```python
from build123d import *

# Parameters (mm, degrees)
F0_W     = 50
F0_H     = 50
F1_DEPTH = 50
F2_R     = 12.5
F3_DEPTH = 213.370338
F4_R     = 10
F5_R     = 12.5
F6_DEPTH = 50
F7_R     = 12.5
F8_DEPTH = 50


with BuildPart() as f1:
    # F0 (on Top) → F1 (new body)
    with BuildSketch(Plane.XY):
        Rectangle(F0_W, F0_H)
    extrude(amount=F1_DEPTH)

    # F2 (on Top) → F3 (cut)
    with BuildSketch(Plane.XY):
        Circle(F2_R)
    extrude(amount=F3_DEPTH, mode=Mode.SUBTRACT)

    # F4
    f4_edges = [f1.edges().sort_by_distance(p)[0] for p in [
        (25, -25, 25),
        (25, 0, 50),
        (25, 25, 25),
        (25, 0, 0),
        (0, 25, 50),
        (0, -25, 50),
        (-25, 0, 50),
        (-25, -25, 25),
        (0, -25, 0),
        (-25, 0, 0),
        (0, 25, 0),
        (-25, 25, 25),
    ]]
    fillet(f4_edges, radius=F4_R)

    # F5 (on Right) → F6 (cut, symmetric)
    with BuildSketch(Plane.YZ):
        with Locations((0, 25)):
            Circle(F5_R)
    extrude(amount=F6_DEPTH, both=True, mode=Mode.SUBTRACT)

    # F7 (on Front) → F8 (cut, symmetric)
    with BuildSketch(Plane.XZ):
        with Locations((0, 25)):
            Circle(F7_R)
    extrude(amount=F8_DEPTH, both=True, mode=Mode.SUBTRACT)


solid = f1.part
```
Build history of the part. All positions in model axes, mm. Round coordinates to 2 decimals unless told otherwise and drop trailing zeros. Loops run counter-clockwise (first coordinate to the right, second up) from the corner with the lowest first, then second, coordinate; pieces in that order, holes last.
Item 1: Saw through at C-C (x = -18.5). List the corners of the cut face in (y, z) (1 decimal).
Item 2: Two-plate mould, pull along Y, no slides. Class faces 1 (the face through (18.83, -9.21, 33.45)), 2 (the face through (0.21, -22.15, 3.01)), 3 (the face through (-14, 0, 50)): released by +Y, released by -Y, zero draft, split by the parting line, or undercut.
Item 3: Saw through at D-D (z = 47). List the corners of the cut face in (x, y), then the cut area to 3 significant figures.
Item 4: Drill centre lines: line 1 along Z through (x, y) = (13, 0); line 2 along X through (y, z) = (-15, 25); line 3 along X through (y, z) = (2, 9). Where is each one in solid material? Low to high.
Item 5: Pin check, flat tips, straight feed: P1, Ø22.5, axis at x = 0, y = 0, coming from the +Z side; P2, Ø1, axis at x = -18.5, y = 3.5, coming from the -Z side. Stop position of each tip, or through.
Item 6: Saw through at A-A (y = 0). List the corners of the cut face in (x, z), then the cut area to 3 significant figures.
Worked answers:
1. outline: (-24.4, 10) arc R9.4 ccw to (-15, 0.6) - (15, 0.6) arc R9.4 ccw to (24.4, 10) - (24.4, 40) arc R9.4 ccw to (15, 49.4) - (-15, 49.4) arc R9.4 ccw to (-24.4, 40) - close; hole circle Ø25 at (0, 25)
2. face 1: undercut
2. face 2: released by -Y
2. face 3: zero draft
3. outline: (-22.14, -15) arc R7.14 ccw to (-15, -22.14) - (15, -22.14) arc R7.14 ccw to (22.14, -15) - (22.14, 15) arc R7.14 ccw to (15, 22.14) - (-15, 22.14) arc R7.14 ccw to (-22.14, 15) - close; hole circle Ø25 at (0, 0)
3. area: 1,430 mm2
4. line 1: z = 0 to 12.5, 37.5 to 50
4. line 2: x = -25 to -12.5, 12.5 to 25
4. line 3: x = -24.95 to -12.34, 12.34 to 24.95
5. P1: passes through
5. P2: stops at z = 0.46
6. outline: (-25, 10) arc R10 ccw to (-15, 0) - (-12.5, 0) - (-12.5, 12.5) - (-25, 12.5) - close; (-25, 37.5) - (-12.5, 37.5) - (-12.5, 50) - (-15, 50) arc R10 ccw to (-25, 40) - close; (12.5, 0) - (15, 0) arc R10 ccw to (25, 10) - (25, 12.5) - (12.5, 12.5) - close; (12.5, 37.5) - (25, 37.5) - (25, 40) arc R10 ccw to (15, 50) - (12.5, 50) - close
6. area: 539 mm2
